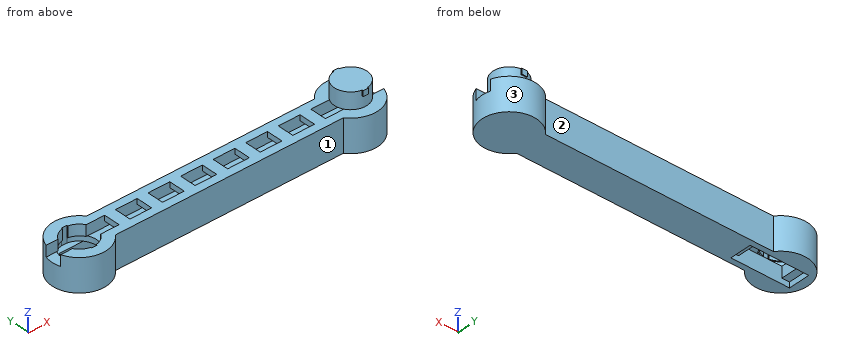
Autodesk Inventor part; units mm, degrees
ref_plane "YZ Plane" through (0, 0, 0) normal (1, 0, 0) x (0, 1, 0)
ref_plane "XZ Plane" through (0, 0, 0) normal (0, 1, 0) x (-1, 0, 0)
ref_plane "XY Plane" through (0, 0, 0) normal (0, 0, 1) x (1, 0, 0)
sketch "Szkic1" plane through (0, 0, 0) normal (0, 0, 1) x (1, 0, 0)
  arc A0 (20, 15) -> (-20, 15) centre (0, 0) ccw
  line L0 (20, 15) -> (125, 15)
  line L1 (125, 15) -> (125, -15)
  line L2 (125, -15) -> (20, -15)
  arc A1 (230, -15) -> (230, 15) centre (250, 0) ccw
  line L3 (230, 15) -> (125, 15)
  line L4 (125, -15) -> (230, -15)
  arc A2 (-20, 15) -> (20, -15) centre (0, 0) ccw
  dimension "d0" = 50
  dimension "d1" = 30
  dimension "d2" = 250
extrude "kształt" add sketch "Szkic1" along normal blind 30
sketch "Szkic2" plane through (0, 0, 30) normal (0, 0, 1) x (1, 0, 0)
  arc A0 (20, 15) -> (20, -15) centre (0, 0) ccw
  line L0 (20, -15) -> (230, -15)
  arc A1 (230, -15) -> (230, 15) centre (250, 0) ccw
  line L1 (230, 15) -> (20, 15)
  line L2 (-23.8485, 7.5) -> (273.8485, 7.5)
  line L3 (273.8485, -7.5) -> (-23.8485, -7.5)
  point P0 (-23.8485, -7.5)
  dimension "d5" = 15
extrude "rowek na kable" cut sketch "Szkic2" against normal blind 10 contours L2 A1 L3 A0
sketch "Szkic3" plane through (0, 0, 30) normal (0, 0, 1) x (1, 0, 0)
  arc A0 (273.8485, 7.5) -> (230, 15) centre (250, 0) ccw
  circle A1 centre (250, 0) radius 15
  point P0 (0, 0)
  dimension "d8" = 30
extrude "odstająćy cosik" add sketch "Szkic3" along normal blind 15
sketch "Szkic4" plane through (0, 0, 30) normal (0, 0, 1) x (1, 0, 0)
  circle A0 centre (0, 0) radius 15
  dimension "d11" = 30
extrude "wgłebiający cosik" cut sketch "Szkic4" against normal blind 15
sketch "Szkic5" plane through (0, 0, 30) normal (0, 0, 1) x (1, 0, 0)
  arc A0 (12.9904, 7.5) -> (-12.9904, 7.5) centre (0, 0) ccw
  line L0 (12.9904, 7.5) -> (237.0096, 7.5)
  arc A1 (262.9904, 7.5) -> (237.0096, 7.5) centre (250, 0) ccw
  line L1 (262.9904, 7.5) -> (273.8485, 7.5)
  arc A2 (273.8485, 7.5) -> (230, 15) centre (250, 0) ccw
  line L2 (230, 15) -> (20, 15)
  arc A3 (20, 15) -> (-23.8485, 7.5) centre (0, 0) ccw
  line L3 (-23.8485, 7.5) -> (-12.9904, 7.5)
  arc A4 (-12.9904, -7.5) -> (12.9904, -7.5) centre (0, 0) ccw
  line L4 (-12.9904, -7.5) -> (-23.8485, -7.5)
  arc A5 (-23.8485, -7.5) -> (20, -15) centre (0, 0) ccw
  line L5 (20, -15) -> (230, -15)
  arc A6 (230, -15) -> (273.8485, -7.5) centre (250, 0) ccw
  line L6 (273.8485, -7.5) -> (262.9904, -7.5)
  arc A7 (237.0096, -7.5) -> (262.9904, -7.5) centre (250, 0) ccw
  line L7 (237.0096, -7.5) -> (12.9904, -7.5)
  line L8 (30, 7.5) -> (40, 7.5)
  line L9 (40, 7.5) -> (40, -7.5)
  line L10 (40, -7.5) -> (30, -7.5)
  line L11 (30, -7.5) -> (30, 7.5)
  arc A8 (-23.8485, -7.5) -> (20, -15) centre (0, 0) ccw
  line L12 (60, -7.5) -> (60, 7.5)
  line L13 (70, 7.5) -> (70, -7.5)
  line L14 (70, -7.5) -> (60, -7.5)
  line L15 (60, 7.5) -> (70, 7.5)
  line L16 (90, -7.5) -> (90, 7.5)
  line L17 (100, 7.5) -> (100, -7.5)
  line L18 (100, -7.5) -> (90, -7.5)
  line L19 (90, 7.5) -> (100, 7.5)
  line L20 (120, -7.5) -> (120, 7.5)
  line L21 (130, 7.5) -> (130, -7.5)
  line L22 (130, -7.5) -> (120, -7.5)
  line L23 (120, 7.5) -> (130, 7.5)
  line L24 (150, -7.5) -> (150, 7.5)
  line L25 (160, 7.5) -> (160, -7.5)
  line L26 (160, -7.5) -> (150, -7.5)
  line L27 (150, 7.5) -> (160, 7.5)
  line L28 (180, -7.5) -> (180, 7.5)
  line L29 (190, 7.5) -> (190, -7.5)
  line L30 (190, -7.5) -> (180, -7.5)
  line L31 (180, 7.5) -> (190, 7.5)
  line L32 (210, -7.5) -> (210, 7.5)
  line L33 (220, 7.5) -> (220, -7.5)
  line L34 (220, -7.5) -> (210, -7.5)
  line L35 (210, 7.5) -> (220, 7.5)
  arc A9 (273.8485, 7.5) -> (230, 15) centre (250, 0) ccw
  line L36 (0, 0) -> (125, 0) construction
  line L37 (125, -7.5) -> (125, 7.5) construction
  line L38 (125, 0) -> (250, 0) construction
  point P0 (70, -7.5)
  point P1 (60, 7.5)
  point P2 (220, -7.5)
  point P3 (210, 7.5)
  point P4 (190, -7.5)
  point P5 (180, 7.5)
  point P6 (160, -7.5)
  point P7 (150, 7.5)
  point P8 (130, -7.5)
  point P9 (120, 7.5)
  point P10 (100, -7.5)
  point P11 (90, 7.5)
  dimension "d15" = 10
  dimension "d18" = 30
extrude "wzmocnienie" add sketch "Szkic5" against normal blind 5 contours L0 L9 L7 L11 | L0 L13 L7 L12 | L0 L17 L7 L16 | L0 L21 L7 L20 | L33 L7 L32 L0 | L0 L25 L7 L24 | L29 L7 L28 L0
sketch "Szkic6" plane through (250, 0, 45) normal (0, 0, 1) x (1, 0, 0)
  circle A0 centre (0, 0) radius 15
  arc A1 (2.5, 15.8035) -> (2.5, -15.8035) centre (0, 0) ccw construction
  line L0 (-2.5, 15.8035) -> (2.5, 15.8035)
  line L1 (2.5, 15.8035) -> (2.5, 14.7902)
  line L2 (2.5, -15.8035) -> (-2.5, -15.8035)
  line L3 (-2.5, -15.8035) -> (-2.5, -14.7902)
  line L4 (2.5, 14.7902) -> (2.5, -14.7902) construction
  line L5 (-2.5, 14.7902) -> (-2.5, 15.8035)
  line L6 (-2.5, -14.7902) -> (-2.5, 14.7902) construction
  line L7 (2.5, -14.7902) -> (2.5, -15.8035)
  point P0 (-250, 0)
  dimension "d25" = 32
  dimension "d27" = 5
extrude "złobek" add sketch "Szkic6" against normal blind 5 contours A0 L5 L0 L1 | L7 L2 L3 A0
sketch "Szkic7" plane through (0, 0, 30) normal (0, 0, 1) x (1, 0, 0)
  circle A0 centre (0, 0) radius 16 construction
  line L0 (-2.5, 15.8035) -> (2.5, 15.8035)
  line L1 (2.5, -15.8035) -> (-2.5, -15.8035)
  arc A1 (12.9904, 7.5) -> (-12.9904, 7.5) centre (0, 0) ccw
  arc A2 (-12.9904, -7.5) -> (12.9904, -7.5) centre (0, 0) ccw
  line L2 (2.5, 15.8035) -> (2.5, 14.7902)
  line L3 (2.5, -14.7902) -> (2.5, -15.8035)
  line L4 (-2.5, -15.8035) -> (-2.5, -14.7902)
  line L5 (-2.5, 14.7902) -> (-2.5, 15.8035)
  arc A3 (2.5, 14.7902) -> (-2.5, 14.7902) centre (0, 0) ccw
  arc A4 (-2.5, -14.7902) -> (2.5, -14.7902) centre (0, 0) ccw
  point P0 (2.5, 15.2968)
  dimension "d30" = 32
  dimension "d32" = 5
extrude "wklęsły żłobek" cut sketch "Szkic7" against normal up to surface (15 mm away)
sketch "Szkic8" plane through (0, 0, 15) normal (0, 0, 1) x (1, 0, 0)
  arc A0 (2.5, -14.7902) -> (2.5, 14.7902) centre (0, 0) ccw
  line L0 (2.5, 15.8035) -> (2.5, 14.7902)
  line L1 (-2.5, 15.8035) -> (2.5, 15.8035)
  line L2 (-2.5, 14.7902) -> (-2.5, 15.8035)
  arc A1 (-2.5, 14.7902) -> (-2.5, -14.7902) centre (0, 0) ccw
  line L3 (-2.5, -15.8035) -> (-2.5, -14.7902)
  line L4 (2.5, -15.8035) -> (-2.5, -15.8035)
  line L5 (2.5, -14.7902) -> (2.5, -15.8035)
  circle A2 centre (0, 0) radius 16
  circle A3 centre (0, 0) radius 15
extrude "rowek" cut sketch "Szkic8" along normal blind 5 contours A0 L0 A2 L5 | L3 A2 L2 A1
sketch "Szkic10" plane through (0, 0, 0) normal (0, 0, -1) x (-1, 0, 0)
  line L0 (10, 10) -> (-30, 10)
  line L1 (-30, 10) -> (-30, -10)
  line L2 (-30, -10) -> (10, -10)
  line L3 (10, -10) -> (10, 10)
  circle A0 centre (0, 0) radius 10 construction
  line L4 (17, 10) -> (-37, 10)
  line L5 (-37, 10) -> (-37, -10)
  line L6 (-37, -10) -> (-30, -10)
  line L7 (17, -10) -> (17, 10)
  line L8 (10, -10) -> (17, -10)
  line L9 (-30, -10) -> (10, -10)
  circle A1 centre (14.5, -5) radius 2.5
  circle A2 centre (14.5, 5) radius 2.5
  line L10 (-10, -10) -> (-10, 10) construction
  circle A3 centre (-34.5, -5) radius 2.5
  circle A4 centre (-34.5, 5) radius 2.5
  point P0 (17, 0)
  point P1 (17, -5)
  point P2 (17, 5)
  point P3 (-37, 5)
  point P4 (-37, -5)
  dimension "d40" = 40
  dimension "d41" = 20
  dimension "d42" = 54
  dimension "d43" = 5
  dimension "d44" = 5
  dimension "d45" = 5
  dimension "d46" = 5
extrude "Wyciągnięcie proste9" cut sketch "Szkic10" against normal blind 15 contours L3 L2 L1 L0
extrude "Wyciągnięcie proste11" cut sketch "Szkic10" against normal blind 5 contours A1 | A2 | L4 L7 L8 L3 | A4 | A3 | L1 L6 L5 L4
properties part number "1stopien" material "Tworzywo sztuczne ABS"
Design review of the part built by this model. Coordinates are the model's own, in mm. Face numbers are marked on the shaded views. A direction names the side the tool comes from. Coordinates: 2 decimals unless noted, no trailing zeros. Write each loop counter-clockwise with the first axis right and the second up, starting at its lowest first coordinate (ties: lowest second). Pieces come first, ordered by that corner, then holes. Notation, with made-up numbers: (-23, -24.5) -> (6, -24.5) arc R7 ccw to (6, -17.5) -> close; hole circle Ø11 at (23.5, 42). An arc over 180 degrees is marked (long way). Write each question's results on one line, items separated by ' | '. Start each with the question number.
(1) Take a section at A-A on x = 34. Write out the cut boundary in (y, z).
(2) Tool access review of the marked faces 1, 2 and 3: name each direction out of +Z, -Z, +X, -X, +Y, -Y from which nothing blocks a thin tool from reaching the whole face with its end or side.
(3) Take a section at D-D on y = 0. Give the number of separate pieces and of enclosed holes in the cut face, and give its area (3 significant figures).
(4) Clearance check with flat-ended pins moving along their axes: P1, Ø5.5, axis at x = 32, y = -3.5, coming from the -Z side; P2, Ø5, axis at y = -7.5, z = 6.5, coming from the +X side; P3, Ø5, axis at y = -1.5, z = 12, coming from the -X side. State where each tip first meets the part, or that it passes through.
(5) Take a section at B-B on x = 0. Write out the cut boundary in (y, z).
(6) For line 1 along Y through (x, z) = (58, 23); line 2 along Z through (x, y) = (92.5, -2); line 3 along X through (y, z) = (20, 21), list the stretches that pass through material, from the lowest coordinate up. Write a range as from..to.
(7) Take a section at C-C on z = 12. Write out the cut boundary in (x, y), and give its area (3 significant figures).
Results found:
1) outline: (-15, 0) -> (-10, 0) -> (-10, 5) -> (10, 5) -> (10, 0) -> (15, 0) -> (15, 30) -> (-15, 30) -> close; hole (-7.5, 20) -> (7.5, 20) -> (7.5, 25) -> (-7.5, 25) -> close
2) face 1: +Z, -Z, -Y | face 2: +Z, -Z, +Y | face 3: +Z, -Z
3) separate pieces: 10 | enclosed holes: 0 | area: 5,970 mm2
4) P1: stops at z = 5 | P2: stops at x = 274.49 | P3: stops at x = -25
5) outline: (-25, 0) -> (-10, 0) -> (-10, 15) -> (-15.8, 15) -> (-15.8, 30) -> (-25, 30) -> close; (10, 0) -> (25, 0) -> (25, 30) -> (15.8, 30) -> (15.8, 15) -> (10, 15) -> close
6) line 1: y = -15..-7.5, 7.5..15 | line 2: z = 0..20, 25..30 | line 3: x = -15..15, 235..265
7) outline: (20, -15) -> (230, -15) arc R25 ccw (long way) to (230, 15) -> (20, 15) arc R25 ccw (long way) to start; hole (-10, -10) -> (30, -10) -> (30, 10) -> (-10, 10) -> close | area: 9,220 mm2
